Can you work these out from the model? Positions are in its coordinate system, mm. Face numbers are marked on the shaded views. Coordinates: 2 decimals unless noted, no trailing zeros. Order: outer loops, then holes, each group sorted by start corner. A loop starts at its lowest first (then second) coordinate and runs counter-clockwise, first axis right, second up. Notation, with made-up numbers: (36, 57) -> (93, 57) arc R28 ccw to (93, 81) -> close; hole circle Ø3 at (-23, -18.75). An arc over 180 degrees is marked (long way). Use a Markdown table: item, result. Add a question column.
1. Suppose I cut it at D-D, the plane z = -19. List the corners of the cut face in (x, y) for me.
2. If I drill on line 1 along Z through (x, y) = (61, 6); line 2 along Z through (x, y) = (18, 1.25); line 3 along X through (y, z) = (0.4, -8.5), over which ranges is the centre line in solid material (lowest first)? Write a range as from..to.
3. Suppose I cut it at A-A, the plane x = 18. List the corners of the cut face in (y, z) for me.
4. For pin 1 Ø2.5 at (x, z) = (18, -8.5) entering from +Y; pin 2 Ø0.8 at (x, y) = (91, 4.5) entering from +Z; pin 3 Ø3 at (x, z) = (90, -28) entering from +Y, each with a flat end and sliding along its axis, tell me the tip position at first contact or that it passes through.
5. We'd pull the mould along Z, two halves only. Please class the marked faces 1 and 2: pulls with the +Z half, pulls with the -Z half, needs draft (parallel to the pull), parting line crosses it, or undercut.
6. Suppose I cut it at B-B, the plane z = -8.5. List the corners of the cut face in (x, y) for me, then the cut area to 3 significant figures.
7. Suppose I cut it at C-C, the plane y = 6. List the corners of the cut face in (x, z) for me.
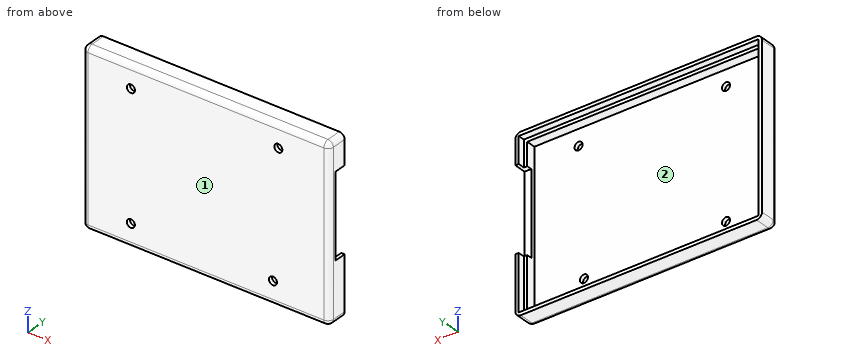
Autodesk Inventor part; units mm, degrees
ref_plane "YZ Plane" through (0, 0, 0) normal (1, 0, 0) x (0, 1, 0)
ref_plane "XZ Plane" through (0, 0, 0) normal (0, 1, 0) x (-1, 0, 0)
ref_plane "XY Plane" through (0, 0, 0) normal (0, 0, 1) x (1, 0, 0)
sketch "Sketch1" plane through (0, 0, 0) normal (0, 1, 0) x (-1, 0, 0)
  line L0 (0, 0) -> (-92, 0)
  line L1 (-92, 0) -> (-92, -64)
  line L2 (-92, -64) -> (0, -64)
  line L3 (0, -64) -> (0, 0)
  dimension "d0" = 64
  dimension "d1" = 92
extrude "Extrusion1" add sketch "Sketch1" along normal blind 7.5
sketch "Sketch2" plane through (0, 7.5, 0) normal (0, 1, 0) x (1, 0, 0)
  line L0 (2.5, 2.5) -> (89.5, 2.5)
  line L1 (89.5, 2.5) -> (89.5, 61.5)
  line L2 (89.5, 61.5) -> (2.5, 61.5)
  line L3 (2.5, 61.5) -> (2.5, 2.5)
  line L4 (0, 64) -> (0, 0)
  line L5 (0, 0) -> (92, 0)
  line L6 (92, 0) -> (92, 64)
  line L7 (92, 64) -> (0, 64)
  dimension "d4" = 2.5
  dimension "d5" = 2.5
  dimension "d6" = 2.5
  dimension "d7" = 2.5
extrude "Extrusion2" cut sketch "Sketch2" against normal blind 6 contours L3 L2 L1 L0
fillet "Fillet1" radius 2 8 edges at (0, 3.75, 0) (46, 0, 0) (92, 3.75, 0) (92, 0, -32) (92, 3.75, -64) (46, 0, -64) (0, 3.75, -64) (0, 0, -32)
sketch "Sketch3" plane through (0, 7.5, 0) normal (0, 1, 0) x (1, 0, 0)
  line L0 (1.25, 1.25) -> (90.75, 1.25)
  line L1 (90.75, 1.25) -> (90.75, 62.75)
  line L2 (90.75, 62.75) -> (1.25, 62.75)
  line L3 (1.25, 62.75) -> (1.25, 1.25)
  line L4 (0, 62) -> (0, 2)
  line L5 (2, 0) -> (90, 0)
  line L6 (92, 2) -> (92, 62)
  line L7 (90, 64) -> (2, 64)
  point P0 (0, 0)
  dimension "d11" = 1.25
  dimension "d12" = 1.25
  dimension "d13" = 1.25
  dimension "d14" = 1.25
extrude "Extrusion3" cut sketch "Sketch3" against normal blind 2.5
sketch "Sketch4" plane through (0, 1.5, 0) normal (0, 1, 0) x (1, 0, 0)
  line L0 (5, 5) -> (87, 5)
  line L1 (87, 5) -> (87, 59) construction
  line L2 (87, 59) -> (5, 59)
  line L3 (5, 59) -> (5, 5)
  line L4 (2.5, 2.5) -> (2.5, 61.5)
  line L5 (89.5, 2.5) -> (2.5, 2.5)
  line L6 (2.5, 61.5) -> (89.5, 61.5)
  line L7 (89.5, 61.5) -> (89.5, 2.5)
  line L8 (18, 55.5) -> (73, 55.5)
  line L9 (73, 55.5) -> (73, 8.5)
  line L10 (73, 8.5) -> (18, 8.5)
  line L11 (18, 8.5) -> (18, 55.5)
  line L12 (71, 55.5) -> (71, 8.5)
  point P0 (0, 0)
  dimension "d17" = 2.5
  dimension "d18" = 2.5
  dimension "d19" = 2.5
  dimension "d20" = 2.5
  dimension "d21" = 14
  dimension "d22" = 13
  dimension "d23" = 54
  dimension "d24" = 82
  dimension "d25" = 3.5
  dimension "d26" = 3.5
  dimension "d44" = 16
  dimension "d45" = 18.5
  dimension "d46" = 16.5
hole "Hole1" at (18, 1.5, -55.5) at (18, 1.5, -8.5) at (73, 1.5, -8.5) at (71, 1.5, -55.5) direction (0, -1, 0) diameter 3 end through all
sketch "Sketch5" plane through (92, 2, -2) normal (1, 0, 0) x (0, 0, -1)
  line L0 (9, 5.5) -> (40, 5.5)
  line L1 (40, 5.5) -> (40, 1)
  line L2 (40, 1) -> (9, 1)
  line L3 (9, 1) -> (9, 5.5)
  line L4 (0, 5.5) -> (60, 5.5)
  line L5 (0, 0) -> (0, 5.5)
  line L6 (60, 5.5) -> (60, 0)
  line L7 (60, 0) -> (0, 0)
  line L8 (59.5, -0.5) -> (0.5, -0.5)
  point P0 (-2, -2)
  dimension "d34" = 0
  dimension "d35" = 9
  dimension "d36" = 20
  dimension "d37" = 4.5
  dimension "d41" = 5.5
  dimension "d42" = 1
  dimension "d43" = 1.5
extrude "Extrusion4" cut sketch "Sketch5" against normal blind 2.5 contours L0 L1 L2 L3
properties part number "hubtest1_3"
Worked out:
| question | item | result |
|---|---|---|
| 1 | outline | (0, 2) arc R2 ccw to (2, 0) -> (90, 0) arc R2 ccw to (92, 2) -> (92, 3) -> (89.5, 3) -> (89.5, 1.5) -> (2.5, 1.5) -> (2.5, 5) -> (1.25, 5) -> (1.25, 7.5) -> (0, 7.5) -> close |
| 2 | line 1 | z = -64..-62.75, -1.25..0 |
| 2 | line 2 | z = -63.85..-57, -54..-10, -7..-0.15 |
| 2 | line 3 | x = 0.8..16.5, 19.5..71.5, 74.5..91.2 |
| 3 | outline | (0, -62) arc R2 ccw to (2, -64) -> (7.5, -64) -> (7.5, -62.75) -> (5, -62.75) -> (5, -61.5) -> (1.5, -61.5) -> (1.5, -57) -> (0, -57) -> close; (0, -54) -> (1.5, -54) -> (1.5, -10) -> (0, -10) -> close; (0, -7) -> (1.5, -7) -> (1.5, -2.5) -> (5, -2.5) -> (5, -1.25) -> (7.5, -1.25) -> (7.5, 0) -> (2, 0) arc R2 ccw to (0, -2) -> close |
| 4 | pin 1 | passes through |
| 4 | pin 2 | stops at z = -0.09 |
| 4 | pin 3 | stops at y = 3 |
| 5 | face 1 | needs draft |
| 5 | face 2 | undercut |
| 6 | outline | (0, 2) arc R2 ccw to (2, 0) -> (16.5, 0) -> (16.5, 1.5) -> (2.5, 1.5) -> (2.5, 5) -> (1.25, 5) -> (1.25, 7.5) -> (0, 7.5) -> close; (19.5, 0) -> (71.5, 0) -> (71.5, 1.5) -> (19.5, 1.5) -> close; (74.5, 0) -> (90, 0) arc R2 ccw to (92, 2) -> (92, 7.5) -> (90.75, 7.5) -> (90.75, 5) -> (89.5, 5) -> (89.5, 1.5) -> (74.5, 1.5) -> close |
| 6 | area | 151 mm² |
| 7 | outline | (0, -62) arc R2 ccw to (2, -64) -> (90, -64) arc R2 ccw to (92, -62) -> (92, -42) -> (90.75, -42) -> (90.75, -62.75) -> (1.25, -62.75) -> (1.25, -1.25) -> (90.75, -1.25) -> (90.75, -11) -> (92, -11) -> (92, -2) arc R2 ccw to (90, 0) -> (2, 0) arc R2 ccw to (0, -2) -> close |
